For this review, take the finished solid that the model builds, in its own axes (mm). A direction names the side the tool comes from. Coordinates: 2 decimals unless noted, no trailing zeros. Loops run counter-clockwise (first coordinate to the right, second up) from the corner with the lowest first, then second, coordinate; pieces in that order, holes last. Notation, with made-up numbers: (10.25, 40.25) - (18.25, 40.25) arc R26 cw to (18.25, 61.25) - close; hole circle Ø10 at (-34.5, -20.5). An arc over 180 degrees is marked (long way). Use one line per item in the form item = value. Start each with the question number.
1. Add section A-A on x = -49.5. Give the boundary of the cut face in (y, z) (3 decimals), and give its area (3 significant figures).
2. For pin 1 Ø3 at (y, z) = (9.5, 27) entering from +X; pin 2 Ø1.5 at (y, z) = (-5, 11.5) entering from -X; pin 3 Ø5 at (x, y) = (-51.5, 11.5) entering from -Z, all flat-tipped, find the tip position at first contact; note any pin that passes through.
3. Machinability: for faces 5 (the face through (-8.897, 3.61, -3.439)), 6 (the face through (-6.35, 10, 2)), which of the approach directions +Z, -Z, +X, -X, +Y, -Y give a long, thin tool a straight path to every point of the face, cutting with its end or side? Answer none if there is none.
4. Draft analysis for pull direction Y (two halves, no side actions). For faces 1 (the face through (-8.985, -3.456, 3.439)), 2 (the face through (-81.234, 6.219, -8.111)), 3 (the face through (-6.35, -9, 3)), 4 (the face through (-8.985, -3.456, -3.439)), state which applies: +Y half, -Y half, draft (parallel to the pull), parting line (faces both ways), or undercut.
5. To check wall thickness, follow probe 1 along Y at (x, z) = (-50, 20.5); probe 2 along Z at (x, y) = (-63, 0.5); probe 3 along Z at (x, y) = (-38.5, 23). State the ranges of each line that lie inside material, in increasing order.
6. Add section B-B on x = -34. Give the boundary of the cut face in (y, z) (3 decimals), and give its area (3 significant figures).
```python
from build123d import *


with BuildPart() as f1:
    # F0 (on Front) → F1 (revolve)
    with BuildSketch(Plane.XZ):
        Polygon((-6.35, 0), (-6.35, 12.7), (-12.7, 0), align=None)
        Polygon((-12.7, 0), (-6.35, 12.7), (-56.4411745648, 37.7455872824), (-90.4398604321, 0), align=None)
    revolve(axis=Axis((-6.35, 0, 0), (1, 0, 0)))

    # F2 (on Top) → F7 section 0
    with BuildSketch(Plane.XY, mode=Mode.PRIVATE) as f7_s0:
        Polygon((-6.35, -10.9985226281), (6.35, -10.9985226281), (12.7, 0), (6.35, 10.9985226281), (-6.35, 10.9985226281), (-12.7, 0), align=None)
    loft([Vertex(0, 0, -25.4), f7_s0.sketch], mode=Mode.SUBTRACT)

    # F2 (on Top) → F8 section 0
    with BuildSketch(Plane.XY, mode=Mode.PRIVATE) as f8_s0:
        Polygon((-6.35, -10.9985226281), (6.35, -10.9985226281), (12.7, 0), (6.35, 10.9985226281), (-6.35, 10.9985226281), (-12.7, 0), align=None)
    loft([Vertex(0, 0, 25.4), f8_s0.sketch], mode=Mode.SUBTRACT)


solid = f1.part
```
Conclusion:
q1.outline = circle Ø68.55 at (0, 0)
q1.area = 3,690 mm^2
q2.pin_1 = -35.2
q2.pin_2 = -79.82
q2.pin_3 = -34.88
q3.face_5 = +X
q3.face_6 = +Z, -Z, +X, +Y, -Y
q4.face_1 = undercut
q4.face_2 = parting line
q4.face_3 = draft
q4.face_4 = undercut
q5.probe_1 = -27.78 to 27.78
q5.probe_2 = -30.46 to 30.46
q5.probe_3 = -17.29 to 17.29
q6.outline = circle Ø53.05 at (0, 0)
q6.area = 2,210 mm^2
